```python
from build123d import *

# Parameters (mm, degrees)
SKIZZE1_R                       = 3.5
SKIZZE1_R_2                     = 1
SKIZZE1_R_3                     = 2
AUFSATZ_LINEAR_AUSTRAGEN1_DEPTH = 3
VERRUNDUNG1_R                   = 5
SKIZZE2_R                       = 12.5
SKIZZE2_R_2                     = 10
AUFSATZ_LINEAR_AUSTRAGEN2_DEPTH = 10
SKIZZE3_R                       = 2
AUFSATZ_LINEAR_AUSTRAGEN3_DEPTH = 5
VERRUNDUNG2_R                   = 1


with BuildPart() as part:
    # Skizze1 → Aufsatz-Linear austragen1 (new body)
    with BuildSketch(Plane.XY):
        with BuildLine():
            ThreePointArc((0, 20), (-20, 0), (0, -20))
            Line((0, -20), (40, -20))
            Line((40, -20), (40, 20))
            Line((40, 20), (0, 20))
        make_face()
        with Locations((21, 0)):
            Circle(SKIZZE1_R, mode=Mode.SUBTRACT)
        Circle(SKIZZE1_R_2, mode=Mode.SUBTRACT)
        with Locations((35, 15)):
            Circle(SKIZZE1_R_3, mode=Mode.SUBTRACT)
        with Locations((35, -15)):
            Circle(SKIZZE1_R_3, mode=Mode.SUBTRACT)
    extrude(amount=AUFSATZ_LINEAR_AUSTRAGEN1_DEPTH)

    # Verrundung1
    verrundung1_edges = [part.edges().sort_by_distance(p)[0] for p in [
        (40, 20, 1.5),
        (40, -20, 1.5),
    ]]
    fillet(verrundung1_edges, radius=VERRUNDUNG1_R)

    # Skizze2 → Aufsatz-Linear austragen2 (add)
    # profile 1 of 3: a face of its own
    with BuildSketch(Plane.XY.offset(3)):
        with Locations((21, 0)):
            Circle(SKIZZE2_R)
        with Locations((21, 0)):
            Circle(SKIZZE2_R_2, mode=Mode.SUBTRACT)
    # profile 2 of 3: a face of its own
    with BuildSketch(Plane.XY.offset(3)):
        with BuildLine():
            Line((21, -7.75), (14.68038767, -7.75))
            ThreePointArc((14.68038767, -7.75), (21, -10), (27.31961233, -7.75))
            Line((27.31961233, -7.75), (21, -7.75))
        make_face()
    # profile 3 of 3: a face of its own
    with BuildSketch(Plane.XY.offset(3)):
        with BuildLine():
            ThreePointArc((27.31961233, 7.75), (21, 10), (14.68038767, 7.75))
            Line((14.68038767, 7.75), (21, 7.75))
            Line((21, 7.75), (27.31961233, 7.75))
        make_face()
    extrude(amount=AUFSATZ_LINEAR_AUSTRAGEN2_DEPTH)

    # Skizze3 → Aufsatz-Linear austragen3 (add)
    with BuildSketch(Plane.XY.offset(3)):
        Circle(SKIZZE3_R)
    extrude(amount=AUFSATZ_LINEAR_AUSTRAGEN3_DEPTH)

    # Verrundung2
    verrundung2_edges = [part.edges().sort_by_distance(p)[0] for p in [
        (-2, 0, 8),
    ]]
    fillet(verrundung2_edges, radius=VERRUNDUNG2_R)


solid = part.part
```
The listing builds one solid part. Answer for the finished solid, in the listing's coordinates (mm). A direction names the side the tool comes from. Give positions to 0.01 mm unless a question says otherwise; leave off trailing zeros. Loops run counter-clockwise (first coordinate to the right, second up) from the corner with the lowest first, then second, coordinate; pieces in that order, holes last. Notation, with made-up numbers: M -30.75,-35.75 L 12.25,-35.75 A31 cw 12.25,-9.75 Z; hole C 9.25,7 d11. An arc over 180 degrees is marked long. One line per item, written item: value.
1. Each of these flat-tipped pins is pushed along its axis until it touches: P1, Ø3, axis at y = 15.5, z = 3.5, coming from the -X side; P2, Ø6, axis at y = 3.5, z = 2.5, coming from the -X side; P3, Ø2, axis at x = 0.5, y = 0, coming from the +Z side. Where does it stop, or does it pass through?
Found:
P1: x = -14.2
P2: x = -19.99
P3: z = 8
2. For a pull along X with two mould halves and no side action, classify faces 4 (the face through (21, -7.75, 8)), 5 (the face through (-20, 0, 1)), 6 (the face through (0, -1, 1)), 7 (the face through (38, 19, 2)) as pulls with the +X half, pulls with the -X half, needs draft (parallel to the pull), parting line crosses it, or undercut.
Found:
face 4: undercut
face 5: pulls with the -X half
face 6: undercut
face 7: pulls with the +X half
3. For faces 1 (the face through (0, 0, 3)), 2 (the face through (21, 4, 3)), 3 (the face through (17, -20, 1)), determine the directions among +Z, -Z, +X, -X, +Y, -Y from which every point of the face is accessible in a straight line to the end or side of a thin tool.
Found:
face 1: -Z
face 2: +Z
face 3: +Z, -Z, +X, -X, -Y
4. Section D-D on x = 6 is taken. Determine the outline of the cut face in (y, z).
Found:
outline: M -20,0 L 20,0 L 20,3 L -20,3 Z
5. Section C-C on z = 10.25 is taken. Determine the outline of the cut face in (x, y).
Found:
outline: C 21,0 d25; hole M 14.68,-7.75 L 27.32,-7.75 A10 ccw 27.32,7.75 L 14.68,7.75 A10 ccw Z
6. Section A-A on z = 1 is taken. Determine the outline of the cut face in (x, y).
Found:
outline: M 0,-20 L 35,-20 A5 ccw 40,-15 L 40,15 A5 ccw 35,20 L 0,20 A20 ccw Z; hole C 0,0 d2; hole C 21,0 d7; hole C 35,-15 d4; hole C 35,15 d4
7. Find the intervals of material crossed by probe 1 along Y at (x, z) = (35, 0.8); probe 2 along Y at (x, z) = (35.5, 1.5); probe 3 along Y at (x, z) = (21, 2.25), in increasing order.
Found:
probe 1: -20 to -17, -13 to 13, 17 to 20
probe 2: -19.97 to -16.94, -13.06 to 13.06, 16.94 to 19.97
probe 3: -20 to -3.5, 3.5 to 20
8. Section B-B on x = 21 is taken. Determine the outline of the cut face in (y, z), plus the area to 3 significant figures.
Found:
outline: M -20,0 L -3.5,0 L -3.5,3 L -7.75,3 L -7.75,13 L -12.5,13 L -12.5,3 L -20,3 Z; M 3.5,0 L 20,0 L 20,3 L 12.5,3 L 12.5,13 L 7.75,13 L 7.75,3 L 3.5,3 Z
area: 194 mm^2
